For this review, use the dimensioned drawing (mm, ordinates from the lowest corner) and the shaded views. A direction names the side the tool comes from. Round coordinates to 2 decimals unless told otherwise and drop trailing zeros. Write each loop counter-clockwise with the first axis right and the second up, starting at its lowest first coordinate (ties: lowest second). Pieces come first, ordered by that corner, then holes. Notation, with made-up numbers: (59.25, 29) - (81.25, 29) arc R22 cw to (81.25, 37) - close; hole circle Ø11 at (83.25, 89.25). An arc over 180 degrees is marked (long way). Return JSON: item names as keys, results as strings.
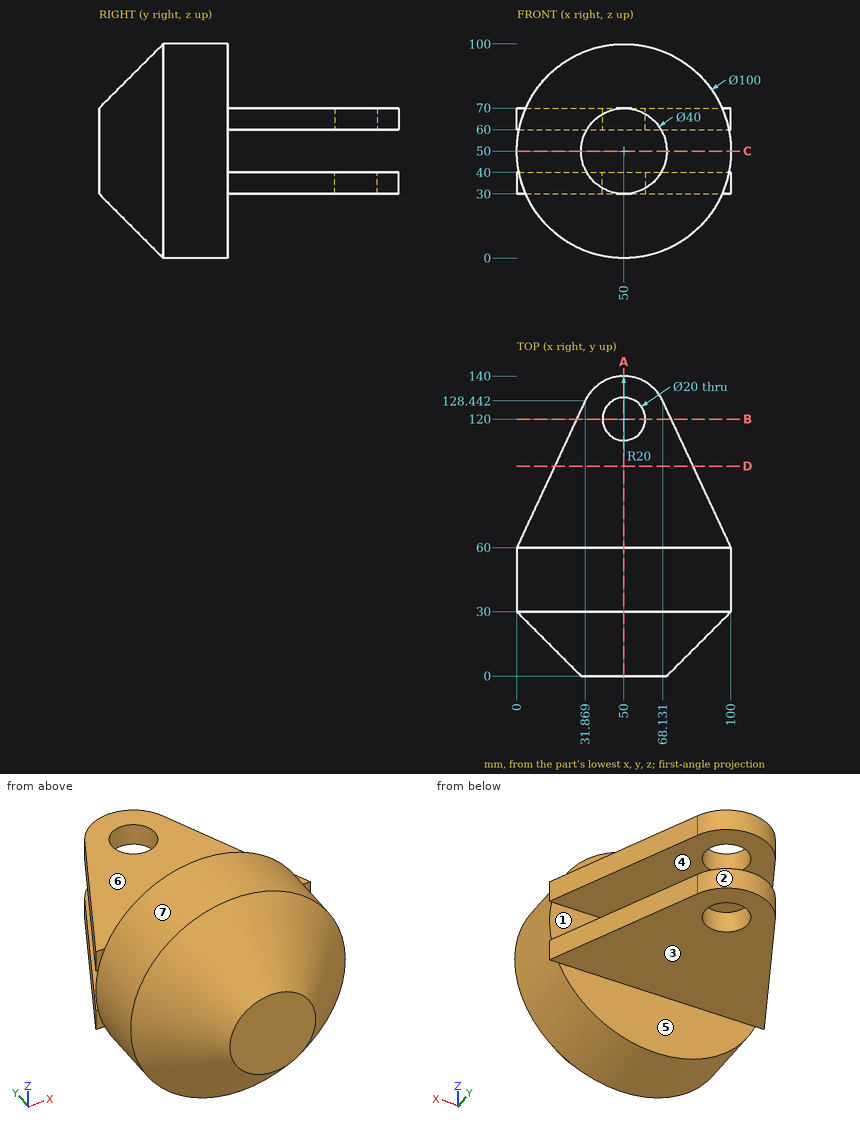
(1) Add section C-C (z = 50). Write out the cut boundary in (x, y), plus the area to 3 significant figures.
Filled in:
{"outline": "(0, 30) - (30, 0) - (70, 0) - (100, 30) - (100, 60) - (0, 60) - close", "area": "5,100 mm2"}
(2) Wall thickness on line 1 (Z direction, x = 66, y = 77); line 2 (Z direction, x = 77.5, y = 12) (1 decimal); line 3 (X direction, y = 23, z = 52) (1 decimal): over which ranges is each line inside the solid? List them lowest first.
Filled in:
{"line 1": "z = 30 to 40, 60 to 70", "line 2": "z = 33.6 to 66.4", "line 3": "x = 7 to 93"}
(3) Add section D-D (y = 98). Write out the cut boundary in (x, z).
Filled in:
{"outline": "(17.69, 30) - (82.31, 30) - (82.31, 40) - (17.69, 40) - close; (17.69, 60) - (82.31, 60) - (82.31, 70) - (17.69, 70) - close"}
(4) Add section A-A (x = 50). Write out the cut boundary in (y, z).
Filled in:
{"outline": "(0, 30) - (30, 0) - (60, 0) - (60, 30) - (110, 30) - (110, 40) - (60, 40) - (60, 60) - (110, 60) - (110, 70) - (60, 70) - (60, 100) - (30, 100) - (0, 70) - close; (130, 30) - (140, 30) - (140, 40) - (130, 40) - close; (130, 60) - (140, 60) - (140, 70) - (130, 70) - close"}
(5) For the marked faces 5, 6 and 7, list the 3-axis set-ups (+Z, -Z, +X, -X, +Y, -Y) from which the entire face can be reached by the end or side of a thin tool; tool diameter is ignored.
Filled in:
{"face 5": "-Z, +X, -X, +Y", "face 6": "+Z, +X, -X, +Y", "face 7": "-Y"}
(6) Clearance check with flat-ended pins moving along their axes: pin 1 Ø1.5 at (x, y) = (35, 123) entering from -Z; pin 2 Ø1.3 at (x, z) = (2.5, 67) entering from -Y; pin 3 Ø15 at (x, z) = (64, 85.5) entering from +Y; pin 4 Ø16 at (x, y) = (50, 120) entering from -Z. State where each tip first meets the part, or that it passes through.
Filled in:
{"pin 1": "stops at z = 30", "pin 2": "stops at y = 29.8", "pin 3": "stops at y = 60", "pin 4": "passes through"}
(7) Mouldability with a two-part tool opening along Z and no side actions: class the marked faces 1, 2, 3 and 4 as released by +Z, released by -Z, zero draft, split by the parting line, or undercut.
Filled in:
{"face 1": "undercut", "face 2": "zero draft", "face 3": "released by -Z", "face 4": "undercut"}
(8) Add section B-B (y = 120). Write out the cut boundary in (x, z).
Filled in:
{"outline": "(27.94, 30) - (40, 30) - (40, 40) - (27.94, 40) - close; (27.94, 60) - (40, 60) - (40, 70) - (27.94, 70) - close; (60, 30) - (72.06, 30) - (72.06, 40) - (60, 40) - close; (60, 60) - (72.06, 60) - (72.06, 70) - (60, 70) - close"}
